```python
from build123d import *

# Parameters (mm, degrees)
F0_W     = 15.8
F0_H     = 15.8
F1_DEPTH = 2
F2_R     = 2.4
F3_DEPTH = 1.8
F4_R     = 0.3


with BuildPart() as f1:
    # F0 (on Top) → F1 (new body)
    with BuildSketch(Plane.XY):
        Rectangle(F0_W, F0_H)
    extrude(amount=F1_DEPTH)

    # F2 (on face) → F3 (join)
    with BuildSketch(Plane.XY.offset(2)):
        with Locations((-4, 4)):
            Circle(F2_R)
        with Locations((4, 4)):
            Circle(F2_R)
    extrude(amount=F3_DEPTH)

    # F4
    f4_edges = [f1.edges().sort_by_distance(p)[0] for p in [
        (1.6, 4, 3.8),
        (-6.4, 4, 3.8),
    ]]
    fillet(f4_edges, radius=F4_R)


solid = f1.part
```
Here's how the part is built. I have some questions about the finished solid (model axes, mm). A direction names the side the tool comes from. Coordinates: 2 decimals unless noted, no trailing zeros. Loops run counter-clockwise (first coordinate to the right, second up) from the corner with the lowest first, then second, coordinate; pieces in that order, holes last. Notation, with made-up numbers: M -7.75,16 L 32.25,16 A24 ccw 32.25,41 Z; hole C 62.25,77.5 d6. An arc over 180 degrees is marked long. One line per item, written item: value.
1. Imagine slicing it at B-B (y = 4). List the corners of the cut face in (x, z) for me.
Geometry says:
outline: M -7.9,0 L 7.9,0 L 7.9,2 L 6.4,2 L 6.4,3.5 A0.3 ccw 6.1,3.8 L 1.9,3.8 A0.3 ccw 1.6,3.5 L 1.6,2 L -1.6,2 L -1.6,3.5 A0.3 ccw -1.9,3.8 L -6.1,3.8 A0.3 ccw -6.4,3.5 L -6.4,2 L -7.9,2 Z
2. Please list where these lines run through material, in increasing order: probe 1 along Z at (x, y) = (0.25, 3); probe 2 along X at (y, z) = (5.25, 2.1); probe 3 along Y at (x, z) = (-5.5, 2.25).
Geometry says:
probe 1: z = 0 to 2
probe 2: x = -6.05 to -1.95, 1.95 to 6.05
probe 3: y = 2.13 to 5.87
3. Thinking about a two-plate mould opening in X: for faces 1 (the cylindrical face through (5.29, 6.024, 2.74)), 2 (the flat face through (0, 7.9, 1)), 3 (the flat face through (-7.9, 0, 1)), 4 (the flat face through (7.9, 0, 1)), which applies, +X half, -X half, draft (parallel to the pull), parting line (faces both ways), or undercut?
Geometry says:
face 1: undercut
face 2: draft
face 3: -X half
face 4: +X half
4. Imagine slicing it at C-C (y = 0.25). List the corners of the cut face in (x, z) for me, and give its area (3 significant figures).
Geometry says:
outline: M -7.9,0 L 7.9,0 L 7.9,2 L -7.9,2 Z
area: 31.6 mm2
5. On a 3-axis mill with a long thin cutter (end or side, diameter ignored), from which of +Z, -Z, +X, -X, +Y, -Y can I reach the whole of each face in a straight line? I mean faces 5 (the cylindrical face through (-2.71, 6.024, 2.74)), 6 (the flat face through (-4, 4, 3.8)). Say none if no direction works.
Geometry says:
face 5: +Z
face 6: +Z, +X, -X, +Y, -Y
6. Imagine slicing it at A-A (x = 4). List the corners of the cut face in (y, z) for me.
Geometry says:
outline: M -7.9,0 L 7.9,0 L 7.9,2 L 6.4,2 L 6.4,3.5 A0.3 ccw 6.1,3.8 L 1.9,3.8 A0.3 ccw 1.6,3.5 L 1.6,2 L -7.9,2 Z
